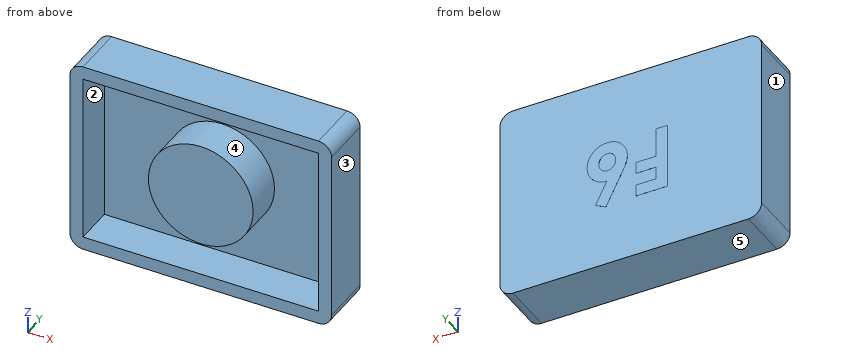
from build123d import *

# Parameters (mm, degrees)
SKETCH1_W           = 12.7
SKETCH1_H           = 9.525
BOSS_EXTRUDE1_DEPTH = 2.54
FILLET1_R           = 0.635
SHELL1_START        = 0.635
SHELL1_OUTLINE_W    = 1.905
SHELL1_OUTLINE_H    = 8.255
SHELL1_DEPTH        = 11.43
SKETCH2_R           = 2.54
BOSS_EXTRUDE2_DEPTH = 1.905
BOSS_EXTRUDE3_DEPTH = 0.00254


# Read off the part's stored shape, not the designer's step: Shell1
with BuildPart() as part:
    # Sketch1 → Boss-Extrude1 (new body)
    with BuildSketch(Plane(origin=(0, 0, 0), x_dir=(1, 0, 0), z_dir=(0, 1, 0))):
        with Locations((6.35, 4.7625)):
            Rectangle(SKETCH1_W, SKETCH1_H)
    extrude(amount=BOSS_EXTRUDE1_DEPTH)

    # Fillet1
    fillet1_edges = [part.edges().sort_by_distance(p)[0] for p in [
        (0, 1.27, -9.525),
        (12.7, 1.27, -9.525),
        (12.7, 1.27, 0),
        (0, 1.27, 0),
    ]]
    fillet(fillet1_edges, radius=FILLET1_R)

    # Shell1 outline → Shell1 (cut)
    with BuildSketch(Plane.YZ.offset(SHELL1_START)):
        with Locations((0.9525, -4.7625)):
            Rectangle(SHELL1_OUTLINE_W, SHELL1_OUTLINE_H)
    extrude(amount=SHELL1_DEPTH, mode=Mode.SUBTRACT)

    # Sketch2 → Boss-Extrude2 (add)
    with BuildSketch(Plane(origin=(0, 1.905, 0), x_dir=(-1, 0, 0), z_dir=(0, -1, 0))):
        with Locations(Location((-6.35, 4.7625, 0), (0, 0, 270))):
            Circle(SKETCH2_R)
    extrude(amount=BOSS_EXTRUDE2_DEPTH)

    # Sketch3 → Boss-Extrude3 (add)
    # profile 1 of 2: a face of its own
    with BuildSketch(Plane(origin=(0, 2.54, 0), x_dir=(1, 0, 0), z_dir=(0, 1, 0))):
        Polygon((4.557346154, 6.477), (6.104141026, 6.477), (6.104141026, 5.907128205), (5.127217949, 5.907128205), (5.127217949, 5.296551282), (6.104141026, 5.296551282), (6.104141026, 4.726679487), (5.127217949, 4.726679487), (5.127217949, 3.302), (4.557346154, 3.302), align=None)
    # profile 2 of 2: a face of its own
    with BuildSketch(Plane(origin=(0, 2.54, 0), x_dir=(1, 0, 0), z_dir=(0, 1, 0))):
        with BuildLine():
            Line((7.556805288, 6.558410256), (8.061167268, 6.30273117))
            Line((8.061167268, 6.30273117), (7.507831931, 5.215141026))
            add(Edge.make_bspline(
                [(7.507831931, 5.215141026), (7.540522464, 5.214294651), (7.604911828, 5.212627578), (7.699647713, 5.199154014), (7.790216983, 5.175861453), (7.877532843, 5.144987227), (7.96052794, 5.103522834), (8.040538956, 5.054198775), (8.115495965, 4.99404278), (8.187117669, 4.92739313), (8.252242916, 4.853554895), (8.308815707, 4.774213367), (8.358117895, 4.691298934), (8.396443432, 4.602956598), (8.427358086, 4.510650736), (8.44966437, 4.41401236), (8.462390729, 4.312761626), (8.46414527, 4.243977417), (8.465038462, 4.208961138)],
                knots=[0, 0, 0, 0, 1.013260694, 1.995783107, 2.958651975, 3.908806537, 4.861209129, 5.829647963, 6.817170299, 7.835534541, 8.860094905, 9.863329007, 10.853101798, 11.844815043, 12.84250023, 13.867713965, 14.914507806, 16, 16, 16, 16], degree=3))
            add(Edge.make_bspline(
                [(8.465038462, 4.208961138), (8.464201467, 4.175207569), (8.462547087, 4.108491238), (8.448871451, 4.010501914), (8.426770904, 3.916486889), (8.395184784, 3.826633922), (8.355036272, 3.740503809), (8.30593736, 3.658147091), (8.24748087, 3.580179194), (8.181177155, 3.507014401), (8.108695756, 3.440324152), (8.032296413, 3.381045977), (7.951331729, 3.332079955), (7.867332031, 3.290727002), (7.778750832, 3.259868741), (7.686913754, 3.236576099), (7.591124371, 3.223135234), (7.526104992, 3.22144503), (7.493203526, 3.220589744)],
                knots=[0, 0, 0, 0, 1.049934834, 2.075270938, 3.072134561, 4.05064612, 5.033440221, 6.024524368, 7.028587226, 8.060776465, 9.092543989, 10.090062252, 11.064205434, 12.031961459, 12.998029633, 13.977230324, 14.976426867, 16, 16, 16, 16], degree=3))
            add(Edge.make_bspline(
                [(7.493203526, 3.220589744), (7.45879859, 3.221291632), (7.391145938, 3.2226718), (7.292153178, 3.238126046), (7.197210601, 3.261390259), (7.1068518, 3.294607602), (7.02051486, 3.336903587), (6.939216244, 3.389240616), (6.862271123, 3.451041549), (6.790499844, 3.520915965), (6.725839271, 3.597453826), (6.668167444, 3.676920054), (6.619377003, 3.759439347), (6.579882279, 3.844923478), (6.54906758, 3.933100047), (6.527626834, 4.024136406), (6.513656209, 4.11779108), (6.512018472, 4.181350442), (6.511192308, 4.213413261)],
                knots=[0, 0, 0, 0, 1.063775006, 2.091769615, 3.092589432, 4.084662827, 5.064601646, 6.061867366, 7.070035304, 8.113879863, 9.156342271, 10.166834137, 11.149076039, 12.117706134, 13.076241869, 14.034148791, 15.008317125, 16, 16, 16, 16], degree=3))
            add(Edge.make_bspline(
                [(6.511192308, 4.213413261), (6.511628837, 4.238242164), (6.512504324, 4.288038176), (6.521302452, 4.362604999), (6.534678698, 4.437367552), (6.550183517, 4.500454562), (6.566148814, 4.553801232), (6.582218008, 4.598947076), (6.602132233, 4.649049092), (6.624897142, 4.70423522), (6.651228609, 4.764439071), (6.680989082, 4.829496544), (6.714252653, 4.899900304), (6.73797416, 4.948256786), (6.750334936, 4.973454327)],
                knots=[0, 0, 0, 0, 1.110454016, 2.227089276, 3.35462975, 4.507227546, 5.131400587, 5.845402449, 6.650387134, 7.543487832, 8.516250726, 9.590168902, 10.744287919, 12, 12, 12, 12], degree=3))
            Line((6.750334936, 4.973454327), (7.556805288, 6.558410256))
        make_face()
        with BuildLine():
            add(Edge.make_bspline(
                [(7.480483173, 4.685974359), (7.45313899, 4.684720139), (7.399630013, 4.682265795), (7.32354825, 4.656562713), (7.254178944, 4.616240974), (7.194048771, 4.560085155), (7.143755415, 4.492976745), (7.106798092, 4.416430641), (7.084566208, 4.331468327), (7.082256458, 4.272064094), (7.081064103, 4.241398037)],
                knots=[0, 0, 0, 0, 0.981744412, 1.921144944, 2.858899012, 3.85339082, 4.86292663, 5.863643845, 6.897155691, 8, 8, 8, 8], degree=3))
            add(Edge.make_bspline(
                [(7.081064103, 4.241398037), (7.082475888, 4.210721768), (7.085221906, 4.151054373), (7.108289737, 4.065283067), (7.146058935, 3.986998689), (7.199027827, 3.919000948), (7.261212545, 3.862557558), (7.330168021, 3.820814972), (7.404744054, 3.795171132), (7.456330117, 3.792042243), (7.482391226, 3.790461538)],
                knots=[0, 0, 0, 0, 1.098279937, 2.136227893, 3.159405121, 4.194678092, 5.206500211, 6.154139736, 7.067477469, 8, 8, 8, 8], degree=3))
            add(Edge.make_bspline(
                [(7.482391226, 3.790461538), (7.509914703, 3.792070396), (7.563893022, 3.795225646), (7.641760287, 3.81979044), (7.7128925, 3.860833701), (7.775787137, 3.917096382), (7.829812434, 3.984318178), (7.867192483, 4.063062388), (7.89132675, 4.149452761), (7.893857997, 4.210062449), (7.895166667, 4.241398037)],
                knots=[0, 0, 0, 0, 0.96921794, 1.900804717, 2.848419905, 3.844199796, 4.861108892, 5.867439427, 6.897452859, 8, 8, 8, 8], degree=3))
            add(Edge.make_bspline(
                [(7.895166667, 4.241398037), (7.893675852, 4.272046189), (7.890788716, 4.331399913), (7.869102903, 4.416760256), (7.830384348, 4.493011323), (7.778953064, 4.560362168), (7.71675353, 4.616492947), (7.644607923, 4.656880703), (7.565050618, 4.682220258), (7.509083321, 4.684704747), (7.480483173, 4.685974359)],
                knots=[0, 0, 0, 0, 1.083229974, 2.097801324, 3.086792542, 4.086858909, 5.079819718, 6.026392613, 6.991456328, 8, 8, 8, 8], degree=3))
        make_face(mode=Mode.SUBTRACT)
    extrude(amount=BOSS_EXTRUDE3_DEPTH)


solid = part.part
Read the model definition and answer for the solid it produces. Units are mm, in the model's axes. Face numbers are marked on the shaded views. A direction names the side the tool comes from. Give positions to 0.01 mm unless a question says otherwise; leave off trailing zeros. Loops run counter-clockwise (first coordinate to the right, second up) from the corner with the lowest first, then second, coordinate; pieces in that order, holes last. Notation, with made-up numbers: (72.25, 60) -> (87.25, 60) arc R16 cw to (87.25, 83) -> close; hole circle Ø2 at (73.25, 17). An arc over 180 degrees is marked (long way). Answer as CSV lines item,"result".
Item 1: Find section D-D on x = 6.35. Give the vertices of the cut face in (y, z) (1 decimal).
Returned:
outline,"(0, -9.5) -> (2.5, -9.5) -> (2.5, 0) -> (0, 0) -> (0, -0.6) -> (1.9, -0.6) -> (1.9, -2.2) -> (0, -2.2) -> (0, -7.3) -> (1.9, -7.3) -> (1.9, -8.9) -> (0, -8.9) -> close"
Item 2: Find section C-C on x = 11.5. Give the vertices of the cut face in (y, z) (3 decimals), plus the area to 3 significant figures.
Returned:
outline,"(0, -9.525) -> (2.54, -9.525) -> (2.54, 0) -> (0, 0) -> (0, -0.635) -> (1.905, -0.635) -> (1.905, -8.89) -> (0, -8.89) -> close"
area,"8.47 mm²"
Item 3: This flat-tipped pin is pushed along its axis until it touches: pin 1 (5 mm diameter, centred on x = 9.5, z = -5, fed in from -Y). Where does it stop, or does it pass through?
Returned:
pin 1,"stops at y = 0"
Item 4: Find section A-A on y = 1.5. State how many separate pieces and enclosed holes the cut face has, plus the area to 3 significant figures.
Returned:
separate pieces,"2"
enclosed holes,"1"
area,"46.5 mm²"
Item 5: Determine the mould class of the marked faces 1, 2 and 3 for opening direction X: +X half, -X half, draft (parallel to the pull), parting line (faces both ways), or undercut.
Returned:
face 1,"-X half"
face 2,"undercut"
face 3,"+X half"
Item 6: Consider line 1 (Z direction, x = 10.25, y = 0.85) (3 decimals); line 2 (X direction, y = 1.15, z = -8) (3 decimals); line 3 (Z direction, x = 8, y = 1.7) (3 decimals). Determine where each line is inside the solid, lowest interval first. Write a range as [from, to].
Returned:
line 1,"z = [-9.525, -8.89], [-0.635, 0]"
line 2,"x = [0, 0.635], [12.065, 12.7]"
line 3,"z = [-9.525, -8.89], [-6.694, -2.831], [-0.635, 0]"
Item 7: Find section B-B on z = -8. Give the vertices of the cut face in (x, y) (3 decimals), plus the area to 3 significant figures.
Returned:
outline,"(0, 0) -> (0.635, 0) -> (0.635, 1.905) -> (12.065, 1.905) -> (12.065, 0) -> (12.7, 0) -> (12.7, 2.54) -> (0, 2.54) -> close"
area,"10.5 mm²"
Item 8: For the marked faces 4 and 5, determine the directions among +Z, -Z, +X, -X, +Y, -Y from which every point of the face is accessible in a straight line to the end or side of a thin tool.
Returned:
face 4,"-Y"
face 5,"-Z, +X, -X, +Y, -Y"
